```python
from build123d import *

# Parameters (mm, degrees)
F1_DEPTH = 25.4
F2_R     = 5.2737089528
F2_R_2   = 6.5522963842
F3_DEPTH = 25.4


with BuildPart() as f1:
    # F0 (on Front) → F1 (new body)
    with BuildSketch(Plane.XZ):
        with BuildLine():
            Line((76.3270024538, 66.4210021496), (-76.3270024538, 66.4210021496))
            ThreePointArc((-76.3270024538, 66.4210021496), (-85.3072585749, 62.7012582707), (-89.0270024538, 53.7210021496))
            Line((-89.0270024538, 53.7210021496), (-89.0270024538, -53.7210021496))
            ThreePointArc((-89.0270024538, -53.7210021496), (-85.3072585749, -62.7012582707), (-76.3270024538, -66.4210021496))
            Line((-76.3270024538, -66.4210021496), (76.3270024538, -66.4210021496))
            ThreePointArc((76.3270024538, -66.4210021496), (85.3072585749, -62.7012582707), (89.0270024538, -53.7210021496))
            Line((89.0270024538, -53.7210021496), (89.0270024538, 53.7210021496))
            ThreePointArc((89.0270024538, 53.7210021496), (85.3072585749, 62.7012582707), (76.3270024538, 66.4210021496))
        make_face()
        with BuildLine():
            ThreePointArc((-83.4389999509, 53.7210021496), (-81.3559441118, 58.7499438076), (-76.3270024538, 60.8329996467))
            Line((-76.3270024538, 60.8329996467), (76.3270024538, 60.8329996467))
            ThreePointArc((76.3270024538, 60.8329996467), (81.3559441118, 58.7499438076), (83.4389999509, 53.7210021496))
            Line((83.4389999509, 53.7210021496), (83.4389999509, -53.7210021496))
            ThreePointArc((83.4389999509, -53.7210021496), (81.3559441118, -58.7499438076), (76.3270024538, -60.8329996467))
            Line((76.3270024538, -60.8329996467), (-76.3270024538, -60.8329996467))
            ThreePointArc((-76.3270024538, -60.8329996467), (-81.3559441118, -58.7499438076), (-83.4389999509, -53.7210021496))
            Line((-83.4389999509, -53.7210021496), (-83.4389999509, 53.7210021496))
        make_face(mode=Mode.SUBTRACT)
    extrude(amount=F1_DEPTH)

    # F2 (on face) → F3 (cut)
    with BuildSketch(Plane.XY.offset(66.4210021496)):
        with BuildLine():
            ThreePointArc((42.4100935748, -17.0894959721), (47.2318985675, -16.44577233), (49.4754982548, -12.1294725306))
            ThreePointArc((49.4754982548, -12.1294725306), (44.2802383376, -6.8563470943), (38.9304142859, -11.9725918196))
            ThreePointArc((38.9304142859, -11.9725918196), (41.455018358, -13.9025059955), (42.4124275114, -16.932615261))
            ThreePointArc((42.4124275114, -16.932615261), (42.411843995, -17.0110642966), (42.4100935748, -17.0894959721))
        make_face()
        with BuildLine():
            ThreePointArc((42.4124275114, -16.932615261), (41.455018358, -13.9025059955), (38.9304142859, -11.9725918196))
            ThreePointArc((38.9304142859, -11.9725918196), (39.8408927075, -15.095039426), (42.4100935748, -17.0894959721))
            ThreePointArc((42.4100935748, -17.0894959721), (42.411843995, -17.0110642966), (42.4124275114, -16.932615261))
        make_face()
        with BuildLine():
            ThreePointArc((42.4100935748, -17.0894959721), (39.8408927075, -15.095039426), (38.9304142859, -11.9725918196))
            ThreePointArc((38.9304142859, -11.9725918196), (32.7778219642, -19.8981821563), (42.4100935748, -17.0894959721))
        make_face()
        with Locations((56.1497411863, -18.1506130663)):
            Circle(F2_R)
        with Locations((25.1907666744, -10.9114747254)):
            Circle(F2_R_2)
        with BuildLine():
            ThreePointArc((1.3571952178, -19.9224330682), (12.2357895359, -19.2440179583), (17.4885247542, -9.6934769201))
            ThreePointArc((17.4885247542, -9.6934769201), (5.8170049948, 1.6094847037), (-5.1057663145, -10.4185817197))
            ThreePointArc((-5.1057663145, -10.4185817197), (1.3158519799, -9.0539178543), (4.9868853689, -14.4966196505))
            ThreePointArc((4.9868853689, -14.4966196505), (3.9957986589, -17.7605935258), (1.3571952178, -19.9224330682))
        make_face()
        with BuildLine():
            ThreePointArc((4.9868853689, -14.4966196505), (1.3158519799, -9.0539178543), (-5.1057663145, -10.4185817197))
            ThreePointArc((-5.1057663145, -10.4185817197), (-3.1716296669, -16.052748164), (1.3571952178, -19.9224330682))
            ThreePointArc((1.3571952178, -19.9224330682), (3.9957986589, -17.7605935258), (4.9868853689, -14.4966196505))
        make_face()
        with BuildLine():
            ThreePointArc((1.3571952178, -19.9224330682), (-3.1716296669, -16.052748164), (-5.1057663145, -10.4185817197))
            ThreePointArc((-5.1057663145, -10.4185817197), (-5.7374792548, -17.7976183831), (1.3571952178, -19.9224330682))
        make_face()
        with Locations((-12.8312785807, -8.4754791148)):
            Circle(F2_R)
        with BuildLine():
            ThreePointArc((-33.6339969355, -12.217504751), (-28.8121919428, -11.5737811089), (-26.5685922555, -7.2574813095))
            ThreePointArc((-26.5685922555, -7.2574813095), (-31.7638521727, -1.9843558732), (-37.1136762245, -7.1006005985))
            ThreePointArc((-37.1136762245, -7.1006005985), (-34.5890721523, -9.0305147744), (-33.6316629989, -12.0606240399))
            ThreePointArc((-33.6316629989, -12.0606240399), (-33.6322465153, -12.1390730755), (-33.6339969355, -12.217504751))
        make_face()
        with BuildLine():
            ThreePointArc((-33.6316629989, -12.0606240399), (-34.5890721523, -9.0305147744), (-37.1136762245, -7.1006005985))
            ThreePointArc((-37.1136762245, -7.1006005985), (-36.2031978028, -10.2230482049), (-33.6339969355, -12.217504751))
            ThreePointArc((-33.6339969355, -12.217504751), (-33.6322465153, -12.1390730755), (-33.6316629989, -12.0606240399))
        make_face()
        with BuildLine():
            ThreePointArc((-33.6339969355, -12.217504751), (-36.2031978028, -10.2230482049), (-37.1136762245, -7.1006005985))
            ThreePointArc((-37.1136762245, -7.1006005985), (-43.2662685461, -15.0261909352), (-33.6339969355, -12.217504751))
        make_face()
        with Locations((-50.8533238359, -6.0394835043)):
            Circle(F2_R)
    extrude(amount=-F3_DEPTH, mode=Mode.SUBTRACT)


solid = f1.part
```
Check sheet for the modelled part. Datum: model origin and axes. Units: mm. A direction names the side the tool comes from. Round coordinates to 2 decimals unless told otherwise and drop trailing zeros. Loops run counter-clockwise (first coordinate to the right, second up) from the corner with the lowest first, then second, coordinate; pieces in that order, holes last. Notation, with made-up numbers: (82.5, 19) -> (123.5, 19) arc R27 cw to (123.5, 57) -> close; hole circle Ø4 at (29.25, 54). An arc over 180 degrees is marked (long way). Answer in a Markdown table with one row per item.
Q1. Go/stop test with a flat-tipped pin: P1, Ø6.5, axis at x = -38.91, y = -12.06, coming from the +Z side. Record where the tip stops, or that it passes through.
Data:
| item | result |
|---|---|
| P1 | stops at z = -60.83 |
Q2. Sectioned sample at C-C on x = -53. Enter the section's corners in (y, z).
Data:
| item | result |
|---|---|
| outline | (-25.4, -66.42) -> (0, -66.42) -> (0, -60.83) -> (-25.4, -60.83) -> close; (-25.4, 60.83) -> (-10.86, 60.83) -> (-10.86, 66.42) -> (-25.4, 66.42) -> close; (-1.22, 60.83) -> (0, 60.83) -> (0, 66.42) -> (-1.22, 66.42) -> close |
Q3. Sectioned sample at A-A on x = -20.5. Enter the section's corners in (y, z).
Data:
| item | result |
|---|---|
| outline | (-25.4, -66.42) -> (0, -66.42) -> (0, -60.83) -> (-25.4, -60.83) -> close; (-25.4, 60.83) -> (0, 60.83) -> (0, 66.42) -> (-25.4, 66.42) -> close |
Q4. Set-up check for faces 4 (the face through (81.3, -12.522, 58.805)), 5 (the face through (-85, -13, -63)), 6 (the face through (-43.37, -14.87, 63.67)): record each of +Z, -Z, +X, -X, +Y, -Y from which the full face is reachable in a straight line by a thin tool's end or side.
Data:
| item | result |
|---|---|
| face 4 | +Y, -Y |
| face 5 | -Z, -X, +Y, -Y |
| face 6 | +Z |
Q5. Sectioned sample at B-B on z = -30. Enter the section's corners in (x, y).
Data:
| item | result |
|---|---|
| outline | (-89.03, -25.4) -> (-83.44, -25.4) -> (-83.44, 0) -> (-89.03, 0) -> close; (83.44, -25.4) -> (89.03, -25.4) -> (89.03, 0) -> (83.44, 0) -> close |
Q6. Release check for a two-part mould opening along X. For faces 1 (the face through (-85, -13, 63)), 2 (the face through (-1, -21, 60.833)), 3 (the face through (89.027, -13, -1)) record: released by +X, released by -X, zero draft, split by the parting line, or undercut.
Data:
| item | result |
|---|---|
| face 1 | released by -X |
| face 2 | undercut |
| face 3 | released by +X |
Q7. Thickness scan on L1, parallel to X at y = -4, z = -28; L2, parallel to Z at x = -21, y = -10.5; L3, parallel to Z at x = -35.5, y = -7.5. Record the ranges inside material, lowest first.
Data:
| item | result |
|---|---|
| L1 | x = -89.03 to -83.44, 83.44 to 89.03 |
| L2 | z = -66.42 to -60.83, 60.83 to 66.42 |
| L3 | z = -66.42 to -60.83 |
